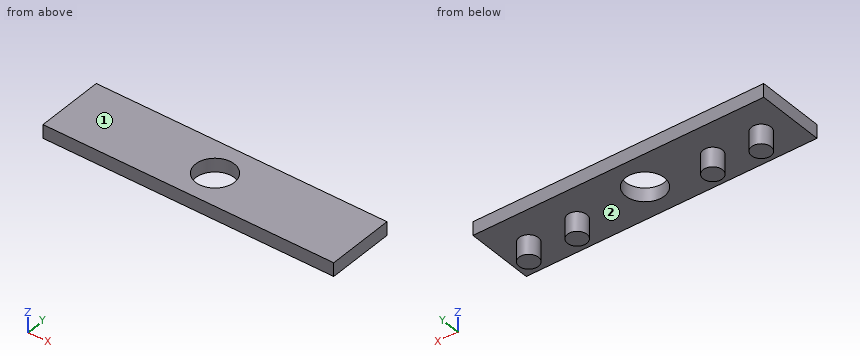
```python
from build123d import *

# Parameters (mm, degrees)
SKETCH1_W           = 150
SKETCH1_H           = 35
SKETCH1_R           = 10
BOSS_EXTRUDE1_DEPTH = 7
SKETCH1_3_R         = 5
BOSS_EXTRUDE2_DEPTH = 10
SCALE1_SCALE        = 0.2
SCALE2_SCALE        = 2


with BuildPart() as part:
    # Sketch1 → Boss-Extrude1 (new body)
    with BuildSketch(Plane.XY):
        Rectangle(SKETCH1_W, SKETCH1_H)
        Circle(SKETCH1_R, mode=Mode.SUBTRACT)
    extrude(amount=BOSS_EXTRUDE1_DEPTH)

    # Sketch1<3> → Boss-Extrude2 (add)
    with BuildSketch(Plane.XY):
        with Locations((60, 0)):
            Circle(SKETCH1_3_R)
        with Locations((35, 0)):
            Circle(SKETCH1_3_R)
        with Locations((-35, 0)):
            Circle(SKETCH1_3_R)
        with Locations((-60, 0)):
            Circle(SKETCH1_3_R)
    extrude(amount=-BOSS_EXTRUDE2_DEPTH)


with BuildPart() as part_1:
    # Scale1: scaled about (0, 0, 2.791541997)
    add(part.part.scale(SCALE1_SCALE).moved(Location((0, 0, 2.233233598))))


with BuildPart() as part_2:
    # Scale2: scaled about (0, 0, 2.791541997)
    add(part_1.part.scale(SCALE2_SCALE).moved(Location((0, 0, -2.791541997))))


solid = part_2.part
```
Geometry check sheet. Reference: the model listing, model coordinates, mm. Face numbers are marked on the shaded views. Coordinates: 2 decimals unless noted, no trailing zeros. Write each loop counter-clockwise with the first axis right and the second up, starting at its lowest first coordinate (ties: lowest second). Pieces come first, ordered by that corner, then holes. Notation, with made-up numbers: M 80,28.5 L 139,28.5 A10 ccw 139,38.5 Z; hole C 38,-31 d9. An arc over 180 degrees is marked long. One line per item, written item: value. Start each with the question number.
(1) Sectioned sample at D-D, the plane x = -24. Enter the section's corners in (y, z).
(2) Scan lines: line 1 along Y through (x, z) = (0, 3.1); line 2 along X through (y, z) = (-1.75, -0.5); line 3 along Z through (x, y) = (-4, 2). Record each from-to range of solid material in increasing order. Write a range as [from, to].
(3) Sectioned sample at A-A, the plane x = 0. Enter the section's corners in (y, z).
(4) Sectioned sample at C-C, the plane y = 0.5. Enter the section's corners in (x, z), and give its area (3 significant figures).
(5) Release check for a two-part mould opening along X. For the marked faces 1 and 2 record: released by +X, released by -X, zero draft, split by the parting line, or undercut.
(6) Depth check by flat-ended pin: pin 1 (1.5 mm diameter, centred on x = 10, y = -0.5, fed in from -Z). Enter the tip coordinate at first touch or a pass-through.
(7) Sectioned sample at B-B, the plane z = 3. Enter the section's corners in (x, y).
Filled sheet:
1. outline: M -7,1.67 L -2,1.67 L -2,-2.33 L 2,-2.33 L 2,1.67 L 7,1.67 L 7,4.47 L -7,4.47 Z
2. line 1: [-7, -4], [4, 7]
2. line 2: [-24.97, -23.03], [-14.97, -13.03], [13.03, 14.97], [23.03, 24.97]
2. line 3: [1.67, 4.47]
3. outline: M -7,1.67 L -4,1.67 L -4,4.47 L -7,4.47 Z; M 4,1.67 L 7,1.67 L 7,4.47 L 4,4.47 Z
4. outline: M -30,1.67 L -25.94,1.67 L -25.94,-2.33 L -22.06,-2.33 L -22.06,1.67 L -15.94,1.67 L -15.94,-2.33 L -12.06,-2.33 L -12.06,1.67 L -3.97,1.67 L -3.97,4.47 L -30,4.47 Z; M 3.97,1.67 L 12.06,1.67 L 12.06,-2.33 L 15.94,-2.33 L 15.94,1.67 L 22.06,1.67 L 22.06,-2.33 L 25.94,-2.33 L 25.94,1.67 L 30,1.67 L 30,4.47 L 3.97,4.47 Z
4. area: 208 mm²
5. face 1: zero draft
5. face 2: undercut
6. pin 1: z = 1.67
7. outline: M -30,-7 L 30,-7 L 30,7 L -30,7 Z; hole C 0,0 d8
